```python
from build123d import *

# Parameters (mm, degrees)
F0_R     = 1.75
F1_DEPTH = 4
F2_W     = 4.25
F2_H     = 40.5
F3_DEPTH = 9
F4_R     = 2.15
F5_DEPTH = 25
F6_R     = 5
F7_W     = 12.1
F7_H     = 4
F8_DEPTH = 1


with BuildPart() as f1:
    # F0 (on Top) → F1 (new body)
    with BuildSketch(Plane.XY):
        with BuildLine():
            Line((18.61898, 20.25), (-6.38102, 20.25))
            ThreePointArc((-6.38102, 20.25), (-10.285671, 17.678153), (-9.464597, 13.075269))
            ThreePointArc((-9.464597, 13.075269), (-4.25, 0), (-9.464597, -13.075269))
            ThreePointArc((-9.464597, -13.075269), (-10.285671, -17.678153), (-6.38102, -20.25))
            Line((-6.38102, -20.25), (18.61898, -20.25))
            Line((18.61898, -20.25), (18.61898, 0))
            Line((18.61898, 0), (18.61898, 20.25))
        make_face()
        with Locations((-6.38102, -16)):
            Circle(F0_R, mode=Mode.SUBTRACT)
        with Locations((-6.38102, 16)):
            Circle(F0_R, mode=Mode.SUBTRACT)
        with BuildLine():
            Line((3.5, 16), (10.86898, 16))
            ThreePointArc((10.86898, 16), (13.343854, 14.974874), (14.36898, 12.5))
            Line((14.36898, 12.5), (14.36898, -12.5))
            ThreePointArc((14.36898, -12.5), (13.343854, -14.974874), (10.86898, -16))
            Line((10.86898, -16), (3.5, -16))
            ThreePointArc((3.5, -16), (1.025126, -14.974874), (0, -12.5))
            Line((0, -12.5), (0, 12.5))
            ThreePointArc((0, 12.5), (1.025126, 14.974874), (3.5, 16))
        make_face(mode=Mode.SUBTRACT)
    extrude(amount=F1_DEPTH)

    # F2 (on face) → F3 (join)
    with BuildSketch(Plane.XY.offset(4)):
        with Locations((16.49398, 0)):
            Rectangle(F2_W, F2_H)
    extrude(amount=F3_DEPTH)

    # F4 (on face) → F5 (cut)
    with BuildSketch(Plane(origin=(14.36898, 0, 0), x_dir=(0, -1, 0), z_dir=(-1, 0, 0))):
        with Locations((0, 8.5)):
            Circle(F4_R)
    extrude(amount=-F5_DEPTH, mode=Mode.SUBTRACT)

    # F6
    f6_edges = [f1.edges().sort_by_distance(p)[0] for p in [
        (16.49398, -20.25, 13),
        (16.49398, 20.25, 13),
    ]]
    fillet(f6_edges, radius=F6_R)

    # F7 (on face) → F8 (join)
    with BuildSketch(Plane.YZ.offset(18.61898)):
        with Locations((-11.2, 8.5)):
            Rectangle(F7_W, F7_H)
        with Locations((11.2, 8.5)):
            Rectangle(F7_W, F7_H)
    extrude(amount=F8_DEPTH)


solid = f1.part
```
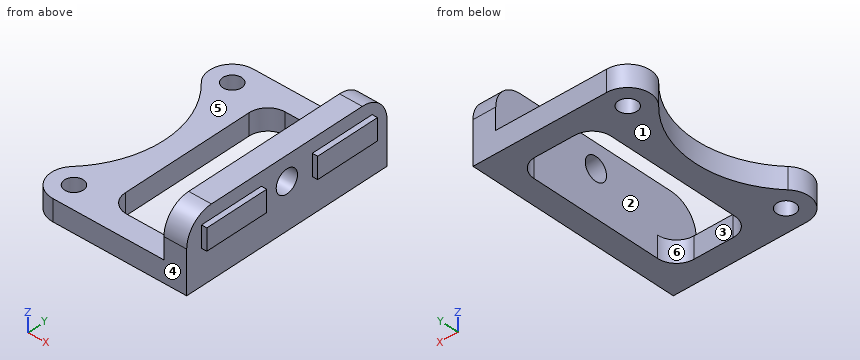
The model under review builds one solid part; all positions refer to its coordinate system, in mm. Face numbers are marked on the shaded views. A direction names the side the tool comes from. Round coordinates to 2 decimals unless told otherwise and drop trailing zeros. Write each loop counter-clockwise with the first axis right and the second up, starting at its lowest first coordinate (ties: lowest second). Pieces come first, ordered by that corner, then holes.
(1) We need section C-C on y = 0. Give the boundary of the cut face in (x, z).
(2) Insertion check: pin 1 (6 mm diameter, centred on x = 0.5, y = 12.5, fed in from -Z); pin 2 (0.5 mm diameter, centred on x = 19, z = 8, fed in from +Y); pin 3 (4 mm diameter, centred on y = 0, z = 6.5, fed in from -X); pin 4 (8 mm diameter, centred on x = -7, y = 5.5, fed in from +Z). Each pin has a flat end and moves straight along its axis. Give the tip position at first contact, or say it passes through.
(3) Machinability: for the marked faces 1, 2 and 3, which of the approach directions +Z, -Z, +X, -X, +Y, -Y give a long, thin tool a straight path to every point of the face, cutting with its end or side? Answer none if there is none.
(4) Wall thickness on L1, parallel to Y at x = 5, z = 0.5; L2, parallel to X at y = -11.5, z = 7.5; L3, parallel to Z at x = 8.5, y = -17: over which ranges is each line inside the solid? List them lowest first.
(5) We need section B-B on z = 3.5. Give the boundary of the cut face in (x, y), and give its area (3 significant figures).
(6) Mouldability with a two-part tool opening along Y and no side actions: class the marked faces 4, 5 and 6 as +Y half, -Y half, draft (parallel to the pull), parting line (faces both ways), or undercut.
(7) We need section A-A on x = 6.5. Give the boundary of the cut face in (y, z), and give its area (3 significant figures).
(8) We need section D-D on x = 17.5. Give the boundary of the cut face in (y, z), and give its area (3 significant figures).
Findings below:
1. outline: (-4.25, 0) - (0, 0) - (0, 4) - (-4.25, 4) - close; (14.37, 0) - (18.62, 0) - (18.62, 6.35) - (14.37, 6.35) - close; (14.37, 10.65) - (18.62, 10.65) - (18.62, 13) - (14.37, 13) - close
2. pin 1: stops at z = 0
2. pin 2: stops at y = 17.25
2. pin 3: stops at x = 14.37
2. pin 4: stops at z = 4
3. face 1: -Z, +X, -X, +Y, -Y
3. face 2: +Z
3. face 3: +Z, -Z
4. L1: y = -20.25 to -16, 16 to 20.25
4. L2: x = 14.37 to 19.62
4. L3: z = 0 to 4
5. outline: (-9.46, -13.08) arc R4.25 ccw to (-6.38, -20.25) - (18.62, -20.25) - (18.62, 20.25) - (-6.38, 20.25) arc R4.25 ccw to (-9.46, 13.08) arc R19 cw to start; hole circle Ø3.5 at (-6.38, -16); hole circle Ø3.5 at (-6.38, 16); hole (0, -12.5) arc R3.5 ccw to (3.5, -16) - (10.87, -16) arc R3.5 ccw to (14.37, -12.5) - (14.37, 12.5) arc R3.5 ccw to (10.87, 16) - (3.5, 16) arc R3.5 ccw to (0, 12.5) - close
5. area: 582 mm2
6. face 4: -Y half
6. face 5: draft
6. face 6: undercut
7. outline: (-20.25, 0) - (-16, 0) - (-16, 4) - (-20.25, 4) - close; (16, 0) - (20.25, 0) - (20.25, 4) - (16, 4) - close
7. area: 34.0 mm2
8. outline: (-20.25, 0) - (20.25, 0) - (20.25, 8) arc R5 ccw to (15.25, 13) - (-15.25, 13) arc R5 ccw to (-20.25, 8) - close; hole circle Ø4.3 at (0, 8.5)
8. area: 501 mm2
